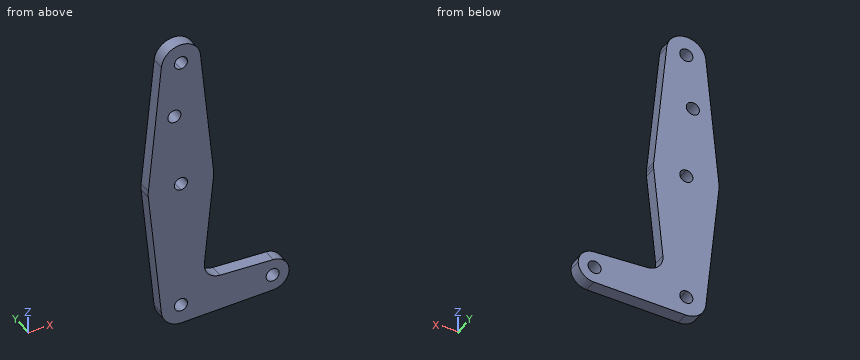
from build123d import *

# Parameters (mm, degrees)
F0_R     = 3.175
F1_DEPTH = 6.35


with BuildPart() as f1:
    # F0 (on Front) → F1 (new body)
    with BuildSketch(Plane.XZ):
        with BuildLine():
            ThreePointArc((9.4772553384, 127.9525), (0, 136.525), (-9.4772553384, 127.9525))
            ThreePointArc((-9.4772553384, 127.9525), (-7.063929059, 120.6104357543), (0, 117.475))
            ThreePointArc((0, 117.475), (6.7351920908, 120.2648079092), (9.525, 127))
            ThreePointArc((9.525, 127), (9.5130563464, 127.4768479324), (9.4772553384, 127.9525))
        make_face()
        with BuildLine():
            ThreePointArc((3.175, 127), (2.2450640303, 124.7549359697), (0, 123.825))
            ThreePointArc((0, 123.825), (-2.2450640303, 129.2450640303), (3.175, 127))
        make_face(mode=Mode.SUBTRACT)
        with BuildLine():
            Line((-9.4772553384, 127.9525), (-15.7954255641, 65.0875))
            ThreePointArc((-15.7954255641, 65.0875), (-10.6492737428, 75.2732150983), (0, 79.375))
            Line((0, 79.375), (0, 100.0252))
            Line((0, 100.0252), (0, 117.475))
            ThreePointArc((0, 117.475), (-7.063929059, 120.6104357543), (-9.4772553384, 127.9525))
        make_face()
        with Locations((-3.175, 100.0252)):
            Circle(F0_R, mode=Mode.SUBTRACT)
        with BuildLine():
            Line((0, 100.0252), (0, 79.375))
            ThreePointArc((0, 79.375), (10.6492737428, 75.2732150983), (15.7954255641, 65.0875))
            Line((15.7954255641, 65.0875), (9.4772553384, 127.9525))
            ThreePointArc((9.4772553384, 127.9525), (9.5130563464, 127.4768479324), (9.525, 127))
            ThreePointArc((9.525, 127), (6.7351920908, 120.2648079092), (0, 117.475))
            Line((0, 117.475), (0, 100.0252))
        make_face()
        with BuildLine():
            ThreePointArc((-15.7954255641, 61.9125), (-10.6492737428, 51.7267849017), (0, 47.625))
            Line((0, 47.625), (0, 60.325))
            ThreePointArc((0, 60.325), (-3.175, 63.5), (0, 66.675))
            Line((0, 66.675), (0, 79.375))
            ThreePointArc((0, 79.375), (-10.6492737428, 75.2732150983), (-15.7954255641, 65.0875))
            ThreePointArc((-15.7954255641, 65.0875), (-15.875, 63.5), (-15.7954255641, 61.9125))
        make_face()
        with BuildLine():
            Line((0, 60.325), (0, 47.625))
            ThreePointArc((0, 47.625), (10.6492737428, 51.7267849017), (15.7954255641, 61.9125))
            ThreePointArc((15.7954255641, 61.9125), (15.8550939106, 62.7052534459), (15.875, 63.5))
            ThreePointArc((15.875, 63.5), (15.8550939106, 64.2947465541), (15.7954255641, 65.0875))
            ThreePointArc((15.7954255641, 65.0875), (10.6492737428, 75.2732150983), (0, 79.375))
            Line((0, 79.375), (0, 66.675))
            ThreePointArc((0, 66.675), (2.2450640303, 65.7450640303), (3.175, 63.5))
            ThreePointArc((3.175, 63.5), (2.2450640303, 61.2549359697), (0, 60.325))
        make_face()
        with BuildLine():
            ThreePointArc((-9.4772553384, -0.9525), (-7.063929059, 6.3895642457), (0, 9.525))
            Line((0, 9.525), (0, 47.625))
            ThreePointArc((0, 47.625), (-10.6492737428, 51.7267849017), (-15.7954255641, 61.9125))
            Line((-15.7954255641, 61.9125), (-9.4772553384, -0.9525))
        make_face()
        with BuildLine():
            Line((0, 47.625), (0, 9.525))
            ThreePointArc((0, 9.525), (6.7351920908, 6.7351920908), (9.525, 0))
            Line((9.525, 0), (36.5125, 0))
            ThreePointArc((36.5125, 0), (38.9384772185, 5.7120069047), (44.7334821429, 7.9324362036))
            Line((44.7334821429, 7.9324362036), (18.9676000005, 8.8532337108))
            ThreePointArc((18.9676000005, 8.8532337108), (13.2611998974, 11.5713591498), (11.3411865923, 17.5933818124))
            Line((11.3411865923, 17.5933818124), (15.7954255641, 61.9125))
            ThreePointArc((15.7954255641, 61.9125), (10.6492737428, 51.7267849017), (0, 47.625))
        make_face()
        with BuildLine():
            ThreePointArc((3.175, 0), (-2.2450640303, -2.2450640303), (0, 3.175))
            Line((0, 3.175), (0, 9.525))
            ThreePointArc((0, 9.525), (-7.063929059, 6.3895642457), (-9.4772553384, -0.9525))
            ThreePointArc((-9.4772553384, -0.9525), (-6.2623833816, -7.1769199091), (0.3401785714, -9.5189234444))
            ThreePointArc((0.3401785714, -9.5189234444), (6.8544082857, -6.6138273378), (9.525, 0))
            Line((9.525, 0), (3.175, 0))
        make_face()
        with BuildLine():
            Line((0, 9.525), (0, 3.175))
            ThreePointArc((0, 3.175), (2.2450640303, 2.2450640303), (3.175, 0))
            Line((3.175, 0), (9.525, 0))
            ThreePointArc((9.525, 0), (6.7351920908, 6.7351920908), (0, 9.525))
        make_face()
        with BuildLine():
            Line((36.5125, 0), (9.525, 0))
            ThreePointArc((9.525, 0), (6.8544082857, -6.6138273378), (0.3401785714, -9.5189234444))
            Line((0.3401785714, -9.5189234444), (44.7334821429, -7.9324362036))
            ThreePointArc((44.7334821429, -7.9324362036), (38.9384772185, -5.7120069047), (36.5125, 0))
        make_face()
        with BuildLine():
            ThreePointArc((44.7334821429, 7.9324362036), (38.9384772185, 5.7120069047), (36.5125, 0))
            ThreePointArc((36.5125, 0), (38.9384772185, -5.7120069047), (44.7334821429, -7.9324362036))
            ThreePointArc((44.7334821429, -7.9324362036), (50.1620069047, -5.5115227815), (52.3875, 0))
            ThreePointArc((52.3875, 0), (50.1620069047, 5.5115227815), (44.7334821429, 7.9324362036))
        make_face()
        with BuildLine():
            ThreePointArc((47.625, 0), (44.45, -3.175), (41.275, 0))
            ThreePointArc((41.275, 0), (44.45, 3.175), (47.625, 0))
        make_face(mode=Mode.SUBTRACT)
    extrude(amount=F1_DEPTH)


solid = f1.part
Geometry check sheet. Reference: the model listing, model coordinates, mm. Give positions to 0.01 mm unless a question says otherwise; leave off trailing zeros. Order: outer loops, then holes, each group sorted by start corner. A loop starts at its lowest first (then second) coordinate and runs counter-clockwise, first axis right, second up.
1) Gauge pin test, flat end, axial feed: pin 1 (3 mm diameter, centred on y = -2.5, z = 63.5, fed in from +X) (3 decimals). Record the tip position at first contact, or that the pin passes through.
Results are:
pin 1: stops at x = 15.875
2) Cross-section at A-A (x = 30). Record the boundary of the cut face in (y, z), then the cut area to 3 significant figures.
Results are:
outline: (-6.35, -8.46) - (0, -8.46) - (0, 8.46) - (-6.35, 8.46) - close
area: 107 mm2
3) Material ranges on probe 1 along Z at (x, y) = (1, -3.75); probe 2 along X at (y, z) = (-3.5, 127) (3 decimals); probe 3 along X at (y, z) = (-4.75, 61.5), recorded low to high.
Results are:
probe 1: z = -9.5 to -3.01, 3.01 to 60.49, 66.51 to 123.99, 130.01 to 136.47
probe 2: x = -9.573 to -3.175, 3.175 to 9.573
probe 3: x = -15.75 to -2.47, 2.47 to 15.75
4) Cross-section at B-B (z = 53). Record the boundary of the cut face in (x, y).
Results are:
outline: (-14.9, -6.35) - (14.9, -6.35) - (14.9, 0) - (-14.9, 0) - close
